Geometry: final body of the model. Coordinates: model frame, mm. A direction names the side the tool comes from. Give positions to 0.01 mm unless a question says otherwise; leave off trailing zeros. Order: outer loops, then holes, each group sorted by start corner. A loop starts at its lowest first (then second) coordinate and runs counter-clockwise, first axis right, second up. Notation, with made-up numbers: (27, -7.5) -> (40, -7.5) arc R14 cw to (40, 5.5) -> close; hole circle Ø6 at (61, 5). An arc over 180 degrees is marked (long way). Answer in a Markdown table with one row per item. Add a question column.
Q1. Cut plane B-B on x = 34. Return the cut outline in (y, z) (1 decimal).
Q2. Cut plane C-C on z = 39.5. Return the cut outline in (x, y), and give its area (3 significant figures).
Q3. Set-up query: faces 5 (the face through (1, -17.462, 43)), 6 (the face through (1, -36, -44.967)), 7 (the face through (1, -9, 77.27)). Return all of +Z, -Z, +X, -X, +Y, -Y with unobstructed straight access to the full face (end or side cutting, diameter ignored); none if empty.
Q4. Line query: line 1 along Z through (x, y) = (39, -37); line 2 along X through (y, z) = (-17, 36.5); line 3 along Z through (x, y) = (12, -25). Output: solid intervals per line, ascending. Write a range as from..to.
Q5. Contact query for flat-ended pins moving along their axis: P1, Ø3.5, axis at x = 8.5, y = -36, coming from the +Z side; P2, Ø6, axis at x = -27, z = -15, coming from the +Y side; P3, Ø4, axis at x = 27, z = -22, coming from the -Y side. Output: stop coordinate, or through.
Q6. Cut plane A-A on y = -32. Return the cut outline in (x, z), and give its area (3 significant figures).
Q7. Pull-direction query (X, two-part tool) for faces 1 (the face through (-15.925, -8.853, 39.981)), 2 (the face through (26.28, -8.85, 33.86)), 3 (the face through (-57.207, -16, -6)), 4 (the face through (60.268, -16, -6)); classes: +X half, -X half, draft (parallel to the pull), parting line (faces both ways), or undercut.
Q8. Cut plane D-D on x = -26.5. Return the cut outline in (y, z) (1 decimal).
from build123d import *

# Parameters (mm, degrees)
F0_W     = 117.475
F0_H     = 68.2625
F1_DEPTH = 41.275
F2_W     = 117.475
F2_H     = 42.8625
F3_DEPTH = 11.1125
F4_W     = 117.475
F4_H     = 17.4625
F5_DEPTH = 66.675
F6_R     = 10.31875
F7_DEPTH = 101.6


with BuildPart() as f1:
    # F0 (on Front) → F1 (new body)
    with BuildSketch(Plane.XZ):
        with Locations((1.530804, -23.5361)):
            Rectangle(F0_W, F0_H)
    extrude(amount=F1_DEPTH)

    # F2 (on face) → F3 (cut)
    with BuildSketch(Plane.XZ.offset(41.275)):
        with Locations((1.530804, -23.5361)):
            Rectangle(F2_W, F2_H)
    extrude(amount=-F3_DEPTH, mode=Mode.SUBTRACT)

    # F4 (on face) → F5 (join)
    with BuildSketch(Plane.XY.offset(10.59515)):
        with Locations((1.530804, -8.73125)):
            Rectangle(F4_W, F4_H)
    extrude(amount=F5_DEPTH)

    # F6 (on face) → F7 (cut)
    with BuildSketch(Plane.XZ.offset(17.4625)):
        with Locations((28.518304, 43.93265)):
            Circle(F6_R)
        with Locations((-25.456696, 43.93265)):
            Circle(F6_R)
    extrude(amount=-F7_DEPTH, mode=Mode.SUBTRACT)


solid = f1.part
Completed:
| question | item | result |
|---|---|---|
| 1 | outline | (-41.3, -57.7) -> (0, -57.7) -> (0, 35.2) -> (-17.5, 35.2) -> (-17.5, 10.6) -> (-41.3, 10.6) -> (-41.3, -2.1) -> (-30.2, -2.1) -> (-30.2, -45) -> (-41.3, -45) -> close; (-17.5, 52.7) -> (0, 52.7) -> (0, 77.3) -> (-17.5, 77.3) -> close |
| 2 | outline | (-57.21, -17.46) -> (-34.77, -17.46) -> (-34.77, 0) -> (-57.21, 0) -> close; (-16.14, -17.46) -> (19.2, -17.46) -> (19.2, 0) -> (-16.14, 0) -> close; (37.84, -17.46) -> (60.27, -17.46) -> (60.27, 0) -> (37.84, 0) -> close |
| 2 | area | 1,400 mm² |
| 3 | face 5 | +Z, +X, -X, -Y |
| 3 | face 6 | +X, -X, -Y |
| 3 | face 7 | +Z, +X, -X, +Y, -Y |
| 4 | line 1 | z = -57.67..-44.97, -2.1..10.6 |
| 4 | line 2 | x = -57.21..-32.61, -18.3..21.36, 35.68..60.27 |
| 4 | line 3 | z = -57.67..10.6 |
| 5 | P1 | stops at z = 10.6 |
| 5 | P2 | stops at y = 0 |
| 5 | P3 | stops at y = -30.16 |
| 6 | outline | (-57.21, -57.67) -> (60.27, -57.67) -> (60.27, -44.97) -> (-57.21, -44.97) -> close; (-57.21, -2.1) -> (60.27, -2.1) -> (60.27, 10.6) -> (-57.21, 10.6) -> close |
| 6 | area | 2,980 mm² |
| 7 | face 1 | undercut |
| 7 | face 2 | undercut |
| 7 | face 3 | -X half |
| 7 | face 4 | +X half |
| 8 | outline | (-41.3, -57.7) -> (0, -57.7) -> (0, 33.7) -> (-17.5, 33.7) -> (-17.5, 10.6) -> (-41.3, 10.6) -> (-41.3, -2.1) -> (-30.2, -2.1) -> (-30.2, -45) -> (-41.3, -45) -> close; (-17.5, 54.2) -> (0, 54.2) -> (0, 77.3) -> (-17.5, 77.3) -> close |
